```python
from build123d import *

# Parameters (mm, degrees)
BOSS_EXTRUDE1_DEPTH      = 135
BOSS_EXTRUDE2_DEPTH      = 36
BOSS_EXTRUDE2_DEPTH_BACK = 36
SKETCH3_W                = 24
SKETCH3_H                = 43.5
CUT_EXTRUDE1_DEPTH       = 178.634456117
SKETCH4_W                = 24
SKETCH4_H                = 42
CUT_EXTRUDE2_DEPTH       = 67.5


with BuildPart() as part:
    # Sketch1 → Boss-Extrude1 (new body)
    with BuildSketch(Plane.XY):
        Polygon((-48, 49.5), (-48, 0), (-25.5, 0), (-25.5, 21), (25.5, 21), (25.5, 0), (48, 0), (48, 49.5), align=None)
    extrude(amount=-BOSS_EXTRUDE1_DEPTH)

    # Sketch2 → Boss-Extrude2 (add, two sides: drawn at the far end of the back side and taken through both)
    with BuildSketch(Plane(origin=(0, 0, 0), x_dir=(0, 0, -1), z_dir=(1, 0, 0)).offset(-BOSS_EXTRUDE2_DEPTH_BACK)):
        with BuildLine():
            Line((37.5, 105), (22.5, 105))
            Line((22.5, 105), (0, 49.5))
            Line((0, 49.5), (135, 49.5))
            Line((135, 49.5), (112.5, 105))
            Line((112.5, 105), (97.5, 105))
            ThreePointArc((97.5, 105), (67.5, 75), (37.5, 105))
        make_face()
    extrude(amount=BOSS_EXTRUDE2_DEPTH + BOSS_EXTRUDE2_DEPTH_BACK)

    # Sketch3 → Cut-Extrude1 (cut, through all)
    with BuildSketch(Plane.XY):
        with Locations((0, 83.25)):
            Rectangle(SKETCH3_W, SKETCH3_H)
    extrude(amount=-CUT_EXTRUDE1_DEPTH, mode=Mode.SUBTRACT)

    # Sketch4 → Cut-Extrude2 (cut)
    with BuildSketch(Plane(origin=(0, 105, 0), x_dir=(1, 0, 0), z_dir=(0, 1, 0))):
        with Locations((36, 66.828706639)):
            Rectangle(SKETCH4_W, SKETCH4_H)
    cut_extrude2 = extrude(amount=-CUT_EXTRUDE2_DEPTH, mode=Mode.SUBTRACT)

    # Mirror1: Cut-Extrude2 across plane
    add(cut_extrude2.mirror(Plane(origin=(0, 0, 0), x_dir=(0, 0, 1), z_dir=(1, 0, 0))), mode=Mode.SUBTRACT)


solid = part.part
```
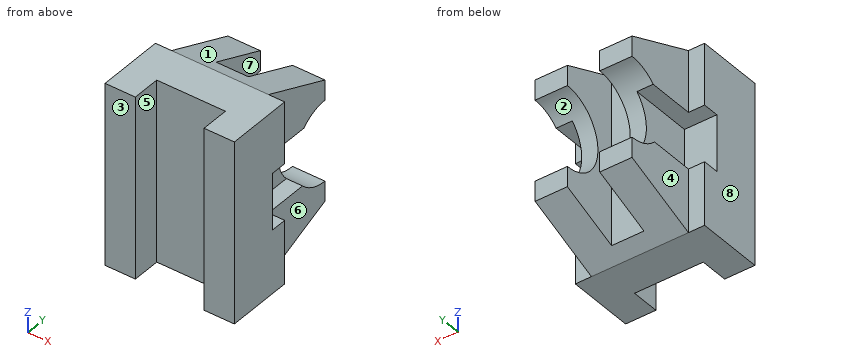
Design review of the part built by this model. Coordinates are the model's own, in mm. Face numbers are marked on the shaded views. A direction names the side the tool comes from. Round coordinates to 2 decimals unless told otherwise and drop trailing zeros. Write each loop counter-clockwise with the first axis right and the second up, starting at its lowest first coordinate (ties: lowest second). Pieces come first, ordered by that corner, then holes.
Item 1: We need section C-C on z = -67.5. Write out the cut boundary in (x, y), and give its area (4 significant figures).
Item 2: Clearance check with flat-ended pins moving along their axes: pin 1 Ø19 at (x, y) = (30.5, 70) entering from +Z; pin 2 Ø8 at (x, y) = (27.5, 67.5) entering from -Z; pin 3 Ø6 at (x, z) = (-39.5, -14) entering from +Y. State where each tip first meets the part, or that it passes through.
Item 3: The part is to be moulded in two halves that separate along Z. For the marked faces 1, 2 and 3, say which applies: +Z half, -Z half, draft (parallel to the pull), parting line (faces both ways), or undercut.
Item 4: We need section A-A on y = 8.5. Write out the cut boundary in (x, z), and give its area (4 significant figures).
Item 5: We need section B-B on x = -4. Write out the cut boundary in (y, z).
Item 6: For probe 1 along X at (y, z) = (6.5, -113); probe 2 along X at (y, z) = (69.5, -28.5); probe 3 along Z at (x, y) = (27, 43), list the stretches that pass through material, from the lowest coordinate up.
Item 7: For the marked faces 4, 5, 6, 7 and 8, list the 3-axis set-ups (+Z, -Z, +X, -X, +Y, -Y) from which the entire face can be reached by the end or side of a thin tool; tool diameter is ignored.
Item 8: We need section D-D on x = 16. Write out the cut boundary in (y, z), and give its area (3 significant figures).
Returned:
1. outline: (-48, 0) - (-25.5, 0) - (-25.5, 21) - (25.5, 21) - (25.5, 0) - (48, 0) - (48, 37.5) - (24, 37.5) - (24, 75) - (12, 75) - (12, 61.5) - (-12, 61.5) - (-12, 75) - (-24, 75) - (-24, 37.5) - (-48, 37.5) - close
1. area: 4,005 mm2
2. pin 1: stops at z = -4.46
2. pin 2: stops at z = -129.32
2. pin 3: stops at y = 49.5
3. face 1: +Z half
3. face 2: undercut
3. face 3: draft
4. outline: (-48, -135) - (-25.5, -135) - (-25.5, 0) - (-48, 0) - close; (25.5, -135) - (48, -135) - (48, 0) - (25.5, 0) - close
4. area: 6,075 mm2
5. outline: (21, -135) - (49.5, -135) - (61.5, -130.14) - (61.5, -4.86) - (49.5, 0) - (21, 0) - close
6. probe 1: x = -48 to -25.5, 25.5 to 48
6. probe 2: x = -36 to -12, 12 to 36
6. probe 3: z = -135 to -87.83, -45.83 to 0
7. face 4: +Z, -Z, -X, +Y
7. face 5: +Z, -Z, -Y
7. face 6: +Z, -Z, +X, +Y
7. face 7: +Z, -Z, +Y
7. face 8: +Z, -Z, -X, +Y, -Y
8. outline: (21, -135) - (49.5, -135) - (105, -112.5) - (105, -97.5) arc R30 cw to (105, -37.5) - (105, -22.5) - (49.5, 0) - (21, 0) - close
8. area: 8,680 mm2
